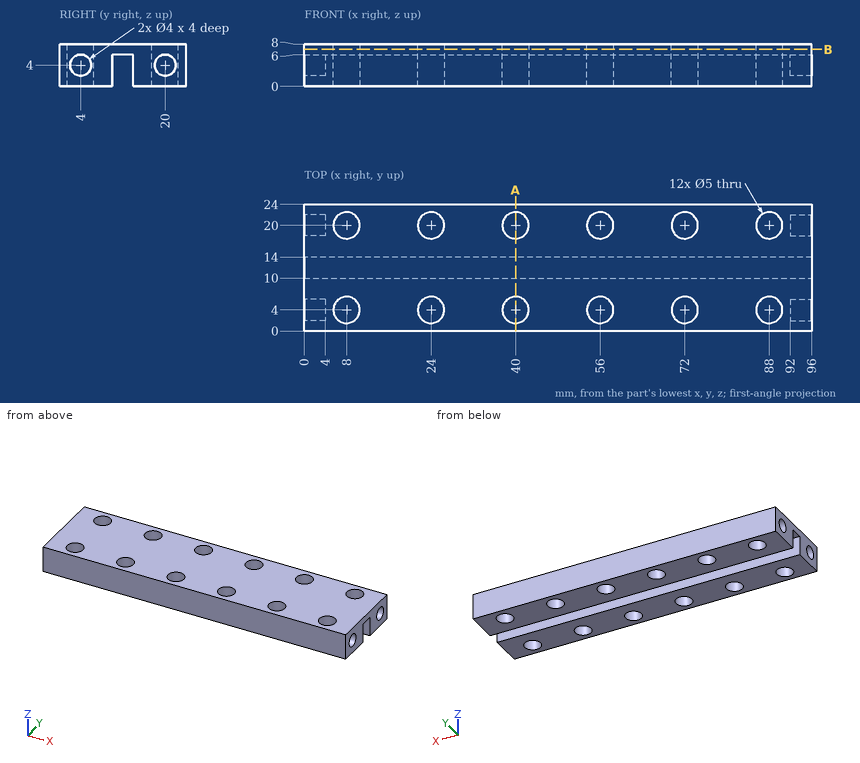
Check sheet for the drawn part. Datum: minimum x, y, z corner. Units: mm. Coordinates: 2 decimals unless noted, no trailing zeros. Loops run counter-clockwise (first coordinate to the right, second up) from the corner with the lowest first, then second, coordinate; pieces in that order, holes last. Notation, with made-up numbers: (-9.5, 85) -> (8.5, 85) arc R25 ccw to (8.5, 99) -> close; hole circle Ø11 at (59, 88.25). An arc over 180 degrees is marked (long way). Answer as a JSON object with one key per item and string values. Group by question number.
Item 1: Scan lines: probe 1 along Y at (x, z) = (94.4, 4); probe 2 along Y at (x, z) = (72, 2.25); probe 3 along Y at (x, z) = (48.5, 5.25). Record each from-to range of solid material in increasing order.
Item 2: Depth check by flat-ended pin: pin 1 (3 mm diameter, centred on x = 44, y = 12, fed in from -Z); pin 2 (2 mm diameter, centred on y = 20, z = 4, fed in from -X). Enter the tip coordinate at first touch or a pass-through.
Item 3: Sectioned sample at A-A on x = 40. Record the boundary of the cut face in (y, z), plus the area to 3 significant figures.
Item 4: Sectioned sample at B-B on z = 7. State how many separate pieces and enclosed holes the cut face has, plus the area to 3 significant figures.
Evaluation:
{
 "1": {"probe 1": "y = 0 to 2, 6 to 10, 14 to 18, 22 to 24", "probe 2": "y = 0 to 1.5, 6.5 to 10, 14 to 17.5, 22.5 to 24", "probe 3": "y = 0 to 10, 14 to 24"},
 "2": {"pin 1": "stops at z = 6", "pin 2": "stops at x = 4"},
 "3": {"outline": "(0, 0) -> (1.5, 0) -> (1.5, 8) -> (0, 8) -> close; (6.5, 0) -> (10, 0) -> (10, 6) -> (14, 6) -> (14, 0) -> (17.5, 0) -> (17.5, 8) -> (6.5, 8) -> close; (22.5, 0) -> (24, 0) -> (24, 8) -> (22.5, 8) -> close", "area": "88.0 mm²"},
 "4": {"separate pieces": "1", "enclosed holes": "12", "area": "2,070 mm²"}
}
